from build123d import *

# Parameters (mm, degrees)
F1_DEPTH = 63.5
F0_W     = 25.402003606
F0_H     = 19.05
F2_DEPTH = 25.4
F3_DEPTH = 15.875
F5_R     = 6.35


with BuildPart() as f1:
    # F0 (on Front) → F1 (new body, symmetric)
    with BuildSketch(Plane.XZ):
        Polygon((22.225, 9.525), (-41.275, 9.525), (-41.275, -9.525), (41.275, -9.525), (41.275, 9.525), align=None)
    extrude(amount=F1_DEPTH, both=True)

    # F0 (on Front) → F2 (join, symmetric)
    with BuildSketch(Plane.XZ):
        with BuildLine():
            Line((22.225, 27.0002), (22.225, 9.525))
            Line((22.225, 9.525), (41.275, 9.525))
            Line((41.275, 9.525), (41.275, 27.0002))
            ThreePointArc((41.275, 27.0002), (45.9246798487, 38.2255201513), (57.15, 42.8752))
            Line((57.15, 42.8752), (60.325, 42.8752))
            Line((60.325, 42.8752), (60.325, 61.9252))
            Line((60.325, 61.9252), (57.15, 61.9252))
            ThreePointArc((57.15, 61.9252), (32.4542956671, 51.6959043329), (22.225, 27.0002))
        make_face()
        with Locations((73.026001803, 52.4002)):
            Rectangle(F0_W, F0_H)
    extrude(amount=F2_DEPTH, both=True)

    # F0 (on Front) → F3 (join)
    with BuildSketch(Plane.XZ):
        with BuildLine():
            add(Edge.make_bspline(
                [(-41.275, 9.525), (-14.1619439489, 32.5014305517), (24.7363013962, 62.9349157899), (57.15, 61.9252)],
                knots=[0, 0, 0, 0, 111.5045361635, 111.5045361635, 111.5045361635, 111.5045361635], degree=3))
            Line((-41.275, 9.525), (22.225, 9.525))
            Line((22.225, 9.525), (22.225, 27.0002))
            ThreePointArc((22.225, 27.0002), (32.4542956671, 51.6959043329), (57.15, 61.9252))
        make_face()
    extrude(amount=F3_DEPTH)

    # F0 (on Front) → F4 (revolve)
    with BuildSketch(Plane.XZ):
        Polygon((85.727003606, 66.675), (85.727003606, 61.9252), (85.727003606, 42.8752), (85.727003606, 38.1), (111.125, 38.1), (111.125, 66.675), align=None)
    revolve(axis=Axis((85.727003606, 0, 52.3875), (0, 0, 1)))

    # F5
    f5_edges = [f1.edges().sort_by_distance(p)[0] for p in [
        (41.275, -63.5, 0),
        (-41.275, -63.5, 0),
        (-41.275, 63.5, 0),
        (41.275, 63.5, 0),
    ]]
    fillet(f5_edges, radius=F5_R)


solid = f1.part
Can you work these out from the model? Positions are in its coordinate system, mm. A direction names the side the tool comes from. Coordinates: 2 decimals unless noted, no trailing zeros. Loops run counter-clockwise (first coordinate to the right, second up) from the corner with the lowest first, then second, coordinate; pieces in that order, holes last. Notation, with made-up numbers: M 42,-24.5 L 64,-24.5 A14 ccw 64,-17.5 Z; hole C 43,11 d9. An arc over 180 degrees is marked long. Answer as CSV lines item,"result". Start each with the question number.
1. Suppose I cut it at A-A, the plane z = 0.5. List the corners of the cut face in (x, y) for me (3 decimals).
2. Suppose I cut it at D-D, the plane x = 100. List the corners of the cut face in (y, z) for me (3 decimals), plus the area to 3 significant figures.
3. If I drill on probe 1 along X at (y, z) = (10, 14.5) (3 decimals); probe 2 along Z at (x, y) = (-32, 37.5) (3 decimals); probe 3 along Z at (x, y) = (72.5, -24), over which ranges is the centre line in solid material (lowest first)? Write a range as [from, to].
4. Suppose I cut it at C-C, the plane y = -47.5. List the corners of the cut face in (x, z) for me (3 decimals).
5. Suppose I cut it at B-B, the plane x = 77. List the corners of the cut face in (y, z) for me (3 decimals), plus the area to 3 significant figures.
6. For faces 1 (the face through (46, 25.4, 42)), 2 (the face through (46, -25.4, 42)), 3 (the face through (32.73, -20.7, 51.97)), 4 (the face through (22.225, 13, 18)), which set-ups out of +Z, -Z, +X, -X, +Y, -Y let a thin tool reach every point of the face, with its end or its side?
7. For pin 1 Ø10 at (x, z) = (92.5, 55.5) entering from +Y; pin 2 Ø5 at (y, z) = (7.5, 18.5) entering from -X (3 decimals); pin 3 Ø1.5 at (x, y) = (-24.5, 30) entering from +Z (3 decimals), each with a flat end and sliding along its axis, tell me the tip position at first contact or that it passes through.
Output:
1,outline,"M -41.275,-57.15 A6.35 ccw -34.925,-63.5 L 34.925,-63.5 A6.35 ccw 41.275,-57.15 L 41.275,57.15 A6.35 ccw 34.925,63.5 L -34.925,63.5 A6.35 ccw -41.275,57.15 Z"
2,outline,"M -21.008,38.1 L 21.008,38.1 L 21.008,66.675 L -21.008,66.675 Z"
2,area,"1,200 mm^2"
3,probe 1,"x = [22.225, 41.275]"
3,probe 2,"z = [-9.525, 9.525]"
3,probe 3,"z = [42.88, 61.93]"
4,outline,"M -41.275,-9.525 L 41.275,-9.525 L 41.275,9.525 L -41.275,9.525 Z"
5,outline,"M -25.4,42.875 L -23.852,42.875 L -23.852,38.1 L 23.852,38.1 L 23.852,42.875 L 25.4,42.875 L 25.4,61.925 L 23.852,61.925 L 23.852,66.675 L -23.852,66.675 L -23.852,61.925 L -25.4,61.925 Z"
5,area,"1,420 mm^2"
6,face 1,"+Z, +X, -X, +Y"
6,face 2,"+Z, +X, -X, -Y"
6,face 3,"+Z, -X, -Y"
6,face 4,"+Z, -X, +Y"
7,pin 1,"stops at y = 25.34"
7,pin 2,"stops at x = 22.225"
7,pin 3,"stops at z = 9.525"
